Design review of the part built by this model. Coordinates are the model's own, in mm. A direction names the side the tool comes from. Coordinates: 2 decimals unless noted, no trailing zeros. Loops run counter-clockwise (first coordinate to the right, second up) from the corner with the lowest first, then second, coordinate; pieces in that order, holes last. Notation, with made-up numbers: (53.25, 82.5) -> (69.25, 82.5) arc R33 ccw to (69.25, 116.5) -> close; hole circle Ø5 at (87.25, -21.5). An arc over 180 degrees is marked (long way). One line per item, written item: value. Start each with the question number.
1. Add section B-B on x = -17.5. Write out the cut boundary in (y, z), plus the area to 3 significant figures.
2. Add section D-D on y = 0. Write out the cut boundary in (x, z), plus the area to 3 significant figures.
3. Add section A-A on y = 62. Write out the cut boundary in (x, z).
4. For probe 1 along X at (y, z) = (34, 16); probe 2 along Y at (x, z) = (-17, -2); probe 3 along X at (y, z) = (-40, 12.5), list the stretches that pass through material, from the lowest coordinate up.
5. Machinability: for faces 1 (the flat face through (-19, -39.7, -0.2)), 2 (the flat face through (-15, -40, -3)), 3 (the cylindrical face through (-0.36, -4.88, 1.08)), 4 (the flat face through (-12.972, 18.226, -7.118)), 5 (the cylindrical face through (20.324, 3.755, -11.923)), which of the approach directions +Z, -Z, +X, -X, +Y, -Y give a long, thin tool a straight path to every point of the face, cutting with its end or side? Answer none if there is none.
6. Insertion check: pin 1 (2 mm diameter, centred on y = 18, z = 7.5, fed in from -X); pin 2 (2 mm diameter, centred on x = 15.5, z = 10.5, fed in from +Y); pin 3 (2 mm diameter, centred on y = -27.5, z = 2.5, fed in from -X); pin 4 (22 mm diameter, centred on y = 13.5, z = 9, fed in from +X). Each pin has a flat end and moves straight along its axis. Give the tip position at first contact, or say it passes through.
7. Draft analysis for pull direction Z (two halves, no side actions). For faces 6 (the flat face through (-15, 27, 2)), 7 (the flat face through (-16.722, -35.618, 14.414)), 8 (the cylindrical face through (-13, 66, -3)), 9 (the cylindrical face through (13, 66, -3)), state which applies: pulls with the +Z half, pulls with the -Z half, needs draft (parallel to the pull), parting line crosses it, or undercut.
8. Add section C-C on x = 22. Write out the cut boundary in (y, z), plus the area to 3 significant figures.
```python
from build123d import *

# Parameters (mm, degrees)
SKETCH_1_R          = 12.5
SKETCH_1_R_2        = 5
EXTRUDE_1_DEPTH     = 25.5
SKETCH_2_R          = 5
SKETCH_2_R_2        = 4
EXTRUDE_2_DEPTH     = 4
SKETCH_3_R          = 4
EXTRUDE_3_DEPTH     = 4
CUT_EXTRUDE_1_DEPTH = 40


with BuildPart() as part:
    # Эскиз1 → Бобышка-Вытянуть1 (new, symmetric)
    with BuildSketch(Plane(origin=(0, 0, 0), x_dir=(0, 0, -1), z_dir=(1, 0, 0))):
        Circle(SKETCH_1_R)
        Circle(SKETCH_1_R_2, mode=Mode.SUBTRACT)
    extrude(amount=EXTRUDE_1_DEPTH, both=True)

    # Эскиз2 → Бобышка-Вытянуть2 (add)
    with BuildSketch(Plane(origin=(11, 0, 0), x_dir=(0, 0, -1), z_dir=(1, 0, 0))):
        with BuildLine():
            Line((19.286048643, -2.880681818), (12.857365762, -45.920454545))
            ThreePointArc((12.857365762, -45.920454545), (0.010828077, -56.99999549), (-12.854148718, -45.94187042))
            Line((-12.854148718, -45.94187042), (-16.017827589, -25))
            Line((-16.017827589, -25), (-23.722142449, 27.142407875))
            ThreePointArc((-23.722142449, 27.142407875), (-23.942938222, 33.992097325), (-22.603459703, 40.713168195))
            Line((-22.603459703, 40.713168195), (-14.279554631, 66.592855272))
            ThreePointArc((-14.279554631, 66.592855272), (6.159605024, 75.676961137), (12.90308202, 54.350786029))
            Line((12.90308202, 54.350786029), (1.079282087, 34.405800714))
            ThreePointArc((1.079282087, 34.405800714), (0.002277121, 25.646156374), (5.709711427, 18.914403089))
            Line((5.709711427, 18.914403089), (8.565518251, 17.518044899))
            ThreePointArc((8.565518251, 17.518044899), (17.261357349, 9.071689063), (19.286048643, -2.880681818))
        make_face()
        Circle(SKETCH_2_R, mode=Mode.SUBTRACT)
        with Locations((0, -44)):
            Circle(SKETCH_2_R_2, mode=Mode.SUBTRACT)
        with Locations((0, 62)):
            Circle(SKETCH_2_R, mode=Mode.SUBTRACT)
    extrude_2 = extrude(amount=EXTRUDE_2_DEPTH)

    # Эскиз3 → Бобышка-Вытянуть3 (add)
    with BuildSketch(Plane(origin=(15, 0, 0), x_dir=(0, 0, -1), z_dir=(1, 0, 0))):
        with BuildLine():
            Line((-16.017827589, -25), (15.982172411, -25))
            Line((15.982172411, -25), (12.857365762, -45.920454545))
            ThreePointArc((12.857365762, -45.920454545), (0.010828077, -56.99999549), (-12.854148718, -45.94187042))
            Line((-12.854148718, -45.94187042), (-16.017827589, -25))
        make_face()
        with Locations((0, -44)):
            Circle(SKETCH_3_R, mode=Mode.SUBTRACT)
    extrude_3 = extrude(amount=EXTRUDE_3_DEPTH)

    # Эскиз5 → Вырез-Вытянуть1 (cut)
    with BuildSketch(Plane.XY.offset(20)):
        Polygon((15, -25), (19, -25), (19, -29), align=None)
        Polygon((15, -57), (15, -29), (11, -25), (11, -57), align=None)
    cut_extrude_1 = extrude(amount=-CUT_EXTRUDE_1_DEPTH, mode=Mode.SUBTRACT)

    # Зеркальное отражение1: Бобышка-Вытянуть2, Бобышка-Вытянуть3, Вырез-Вытянуть1 across plane
    add(extrude_2.mirror(Plane(origin=(0, 0, 0), x_dir=(0, 0, 1), z_dir=(1, 0, 0))))
    add(extrude_3.mirror(Plane(origin=(0, 0, 0), x_dir=(0, 0, 1), z_dir=(1, 0, 0))))
    add(cut_extrude_1.mirror(Plane(origin=(0, 0, 0), x_dir=(0, 0, 1), z_dir=(1, 0, 0))), mode=Mode.SUBTRACT)


solid = part.part
```
Worked answers:
1. outline: (-45.94, 12.85) arc R13 ccw to (-45.92, -12.86) -> (-27.5, -15.61) -> (-27.5, 15.64) -> close; circle Ø25 at (0, 0); hole circle Ø8 at (-44, 0); hole circle Ø10 at (0, 0)
1. area: 1,100 mm²
2. outline: (-25.5, -12.5) -> (-15, -12.5) -> (-15, -19.5) -> (-11, -19.5) -> (-11, -12.5) -> (11, -12.5) -> (11, -19.5) -> (15, -19.5) -> (15, -12.5) -> (25.5, -12.5) -> (25.5, -5) -> (-25.5, -5) -> close; (-25.5, 5) -> (25.5, 5) -> (25.5, 12.5) -> (15, 12.5) -> (15, 19.71) -> (11, 19.71) -> (11, 12.5) -> (-11, 12.5) -> (-11, 19.71) -> (-15, 19.71) -> (-15, 12.5) -> (-25.5, 12.5) -> close
2. area: 879 mm²
3. outline: (-15, -15) -> (-11, -15) -> (-11, -5) -> (-15, -5) -> close; (-15, 5) -> (-11, 5) -> (-11, 15.76) -> (-15, 15.76) -> close; (11, -15) -> (15, -15) -> (15, -5) -> (11, -5) -> close; (11, 5) -> (15, 5) -> (15, 15.76) -> (11, 15.76) -> close
4. probe 1: x = -15 to -11, 11 to 15
4. probe 2: y = -56.85 to -47.46, -40.54 to -27, -12.34 to -4.58, 4.58 to 12.34
4. probe 3: x = -19 to -15, 15 to 19
5. face 1: +Z, -Z, -X, -Y
5. face 2: +Z, -Z, -Y
5. face 3: +X, -X
5. face 4: -Z, +X, -X
5. face 5: +X
6. pin 1: stops at x = -15
6. pin 2: stops at y = 73.5
6. pin 3: stops at x = -18.5
6. pin 4: stops at x = 25.5
7. face 6: needs draft
7. face 7: pulls with the +Z half
7. face 8: undercut
7. face 9: undercut
8. outline: circle Ø25 at (0, 0); hole circle Ø10 at (0, 0)
8. area: 412 mm²
